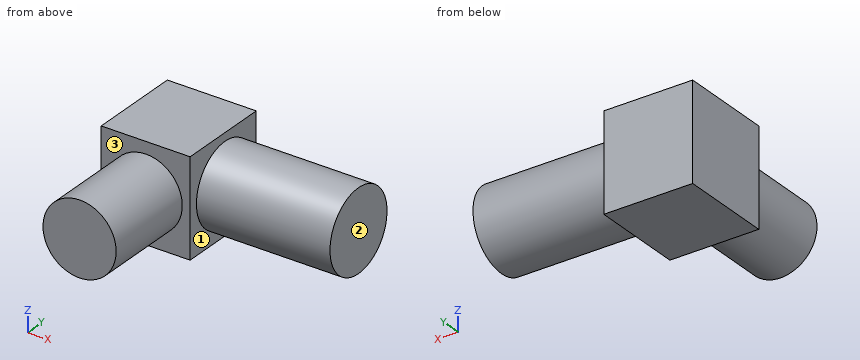
```python
from build123d import *

# Parameters (mm, degrees)
SKETCH1_R           = 21.921131465
BOSS_EXTRUDE1_DEPTH = 56
SKETCH2_W           = 53.266946292
SKETCH2_H           = 58.053682116
BOSS_EXTRUDE2_DEPTH = 56
SKETCH3_R           = 24.156846208
BOSS_EXTRUDE3_DEPTH = 80


with BuildPart() as part:
    # Sketch1 → Boss-Extrude1 (new body)
    with BuildSketch(Plane(origin=(0, 0, 0), x_dir=(1, 0, 0), z_dir=(0, 1, 0))):
        with Locations(Location((0, 0, 0), (0, 0, 270))):
            Circle(SKETCH1_R)
    extrude(amount=BOSS_EXTRUDE1_DEPTH)

    # Sketch2 → Boss-Extrude2 (add)
    with BuildSketch(Plane(origin=(0, 56, 0), x_dir=(1, 0, 0), z_dir=(0, 1, 0))):
        Rectangle(SKETCH2_W, SKETCH2_H)
    extrude(amount=BOSS_EXTRUDE2_DEPTH)

    # Sketch3 → Boss-Extrude3 (add)
    with BuildSketch(Plane(origin=(26.633473146, 0, 0), x_dir=(0, 0, -1), z_dir=(1, 0, 0))):
        with Locations((0, 85.49534666)):
            Circle(SKETCH3_R)
    extrude(amount=BOSS_EXTRUDE3_DEPTH)


solid = part.part
```
Geometry check sheet. Reference: the model listing, model coordinates, mm. Face numbers are marked on the shaded views. A direction names the side the tool comes from. Coordinates: 2 decimals unless noted, no trailing zeros. Loops run counter-clockwise (first coordinate to the right, second up) from the corner with the lowest first, then second, coordinate; pieces in that order, holes last.
Item 1: Sectioned sample at B-B, the plane z = 0. Record the boundary of the cut face in (x, y), then the cut area to 3 significant figures.
Item 2: Access from +Z, -Z, +X, -X, +Y, -Y to the whole of each face (thin tool, end or side, straight path). Record for the marked faces 1, 2 and 3.
Item 3: Sectioned sample at D-D, the plane z = -10. Record the boundary of the cut face in (x, y).
Item 4: Sectioned sample at A-A, the plane x = 0. Record the boundary of the cut face in (y, z), then the cut area to 3 significant figures.
Item 5: Go/stop test with flat-tipped pins: pin 1 Ø5 at (x, z) = (88.5, 6) entering from -Y; pin 2 Ø8 at (x, z) = (86.5, 8.5) entering from +Y; pin 3 Ø10 at (y, z) = (47, -6.5) entering from -X; pin 4 Ø1 at (x, y) = (24, 14) entering from +Z. Record where each tip stops, or that it passes through.
Item 6: Sectioned sample at C-C, the plane y = 79. Record the boundary of the cut face in (x, z), then the cut area to 3 significant figures.
Item 7: Thickness scan on line 1 (X direction, y = 58, z = 25); line 2 (Y direction, x = -19.5, z = -22); line 3 (X direction, y = 7.5, z = -0.5). Record the ranges inside material, lowest first.
Check result:
1. outline: (-26.63, 56) - (-21.92, 56) - (-21.92, 0) - (21.92, 0) - (21.92, 56) - (26.63, 56) - (26.63, 61.34) - (106.63, 61.34) - (106.63, 109.65) - (26.63, 109.65) - (26.63, 112) - (-26.63, 112) - close
1. area: 9,300 mm2
2. face 1: +X
2. face 2: +Z, -Z, +X, +Y, -Y
2. face 3: -Y
3. outline: (-26.63, 56) - (-19.51, 56) - (-19.51, 0) - (19.51, 0) - (19.51, 56) - (26.63, 56) - (26.63, 63.51) - (106.63, 63.51) - (106.63, 107.49) - (26.63, 107.49) - (26.63, 112) - (-26.63, 112) - close
4. outline: (0, -21.92) - (56, -21.92) - (56, -29.03) - (112, -29.03) - (112, 29.03) - (56, 29.03) - (56, 21.92) - (0, 21.92) - close
4. area: 5,710 mm2
5. pin 1: stops at y = 61.59
5. pin 2: stops at y = 109.23
5. pin 3: stops at x = -21.87
5. pin 4: passes through
6. outline: (-26.63, -29.03) - (26.63, -29.03) - (26.63, -23.27) - (106.63, -23.27) - (106.63, 23.27) - (26.63, 23.27) - (26.63, 29.03) - (-26.63, 29.03) - close
6. area: 6,820 mm2
7. line 1: x = -26.63 to 26.63
7. line 2: y = 56 to 112
7. line 3: x = -21.92 to 21.92
